Job drawing, mm, ordinate dimensions from the low corner. One solid piece. A direction names the side the tool comes from. Round coordinates to 2 decimals unless told otherwise and drop trailing zeros. Loops run counter-clockwise (first coordinate to the right, second up) from the corner with the lowest first, then second, coordinate; pieces in that order, holes last.
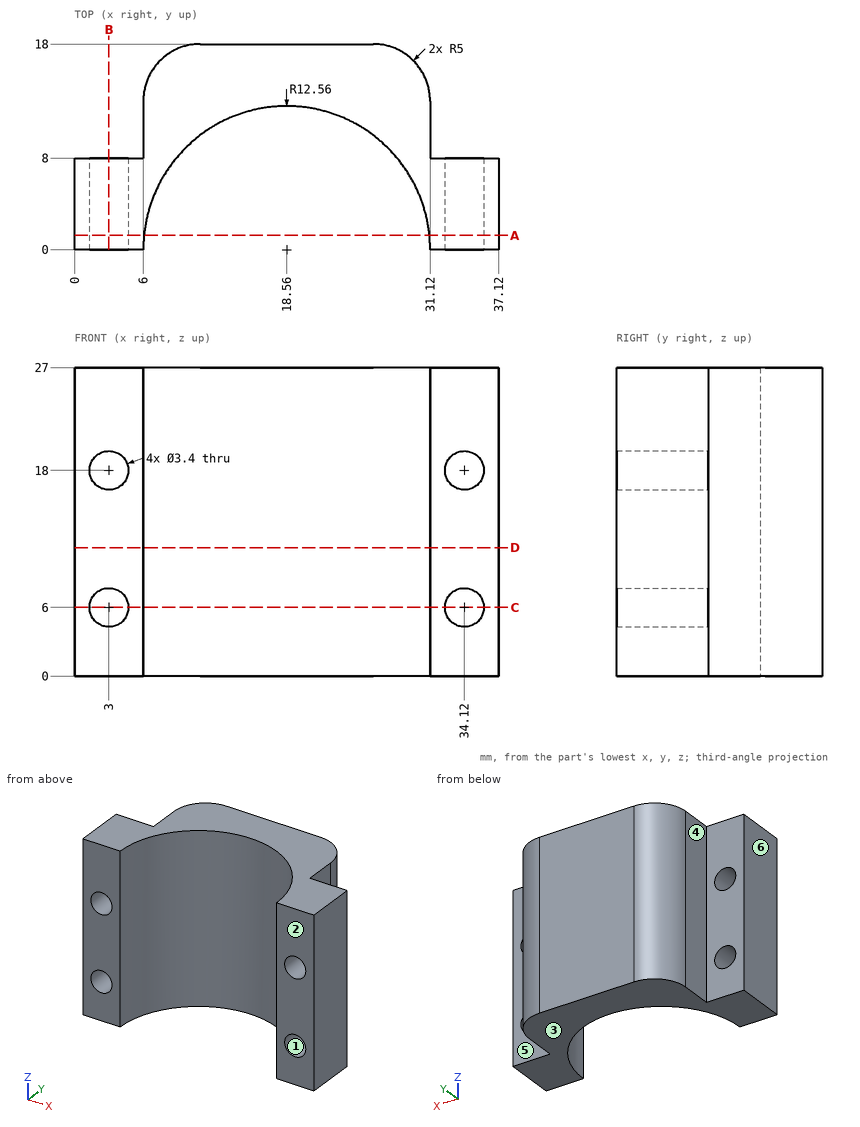
Item 1: Probe line 1 (Z direction, x = 3, y = 5.5); line 2 (X direction, y = 5.5, z = 18); line 3 (X direction, y = 3.5, z = 6). List the from-to ranges inside material, lowest first.
Answers follow:
line 1: z = 0 to 4.3, 7.7 to 16.3, 19.7 to 27
line 2: x = 0 to 1.3, 4.7 to 7.27, 29.85 to 32.42, 35.82 to 37.12
line 3: x = 0 to 1.3, 4.7 to 6.5, 30.62 to 32.42, 35.82 to 37.12
Item 2: Cut at C-C, the plane z = 6. Give the cut face in (x, y).
Answers follow:
outline: (0, 0) - (1.3, 0) - (1.3, 8) - (0, 8) - close; (4.7, 0) - (6, 0) arc R12.56 cw to (31.12, 0) - (32.42, 0) - (32.42, 8) - (31.12, 8) - (31.12, 13) arc R5 ccw to (26.12, 18) - (11, 18) arc R5 ccw to (6, 13) - (6, 8) - (4.7, 8) - close; (35.82, 0) - (37.12, 0) - (37.12, 8) - (35.82, 8) - close
Item 3: 3-axis set-ups, long thin cutter, end or side, ignore diameter. For the marked faces 4, 5 and 6: which of +Z, -Z, +X, -X, +Y, -Y reach the whole face in a straight line?
Answers follow:
face 4: +Z, -Z, -X, +Y
face 5: +Z, -Z, +X, +Y
face 6: +Z, -Z, -X, +Y, -Y
Item 4: Flat gauge pins, fed straight in: P1, Ø4, axis at x = 21, z = 23.5, coming from the -Y side; P2, Ø2, axis at x = 28, z = 8, coming from the +Y side; P3, Ø10, axis at x = 18, z = 11.5, coming from the -Y side. Where does each tip first touch, or does it go through?
Answers follow:
P1: stops at y = 11.75
P2: stops at y = 17.92
P3: stops at y = 11.26
Item 5: Cut at D-D, the plane z = 11.25. Give the cut face in (x, y).
Answers follow:
outline: (0, 0) - (6, 0) arc R12.56 cw to (31.12, 0) - (37.12, 0) - (37.12, 8) - (31.12, 8) - (31.12, 13) arc R5 ccw to (26.12, 18) - (11, 18) arc R5 ccw to (6, 13) - (6, 8) - (0, 8) - close
Item 6: Cut at A-A, the plane y = 1.25. Give the cut face in (x, z), plus the area to 3 significant figures.
Answers follow:
outline: (0, 0) - (6.06, 0) - (6.06, 27) - (0, 27) - close; (31.06, 0) - (37.12, 0) - (37.12, 27) - (31.06, 27) - close; hole circle Ø3.4 at (3, 6); hole circle Ø3.4 at (3, 18); hole circle Ø3.4 at (34.12, 6); hole circle Ø3.4 at (34.12, 18)
area: 291 mm2
Item 7: Two-plate mould, pull along Z, no slides. Class the marked faces 1, 2 and 3: released by +Z, released by -Z, zero draft, split by the parting line, or undercut.
Answers follow:
face 1: undercut
face 2: zero draft
face 3: released by -Z
Item 8: Cut at B-B, the plane x = 3. Give the cut face in (y, z).
Answers follow:
outline: (0, 0) - (8, 0) - (8, 4.3) - (0, 4.3) - close; (0, 7.7) - (8, 7.7) - (8, 16.3) - (0, 16.3) - close; (0, 19.7) - (8, 19.7) - (8, 27) - (0, 27) - close
